CAD build for the part. Positions are in the model's coordinates, mm. A direction names the side the tool comes from. Round coordinates to 2 decimals unless told otherwise and drop trailing zeros. Loops run counter-clockwise (first coordinate to the right, second up) from the corner with the lowest first, then second, coordinate; pieces in that order, holes last.
from build123d import *

# Parameters (mm, degrees)
EXTRUDE_1_DEPTH     = 0.8
SKETCH_2_R          = 1.65
EXTRUDE_2_DEPTH     = 3.18
EXTRUDE_START       = 0.8
EXTRUDE_3_DEPTH     = 0.8
SKETCH_5_R          = 0.81
CUT_EXTRUDE_1_DEPTH = 4.8


with BuildPart() as part:
    # 草图1 → 凸台-拉伸1 (new body)
    with BuildSketch(Plane.XY):
        with BuildLine():
            ThreePointArc((1.190625, 2.753618004), (-3, 0), (1.190625, -2.753618004))
            ThreePointArc((1.190625, -2.753618004), (3.175, -2.342981343), (5.159375, -2.753618004))
            ThreePointArc((5.159375, -2.753618004), (9.35, 0), (5.159375, 2.753618004))
            ThreePointArc((5.159375, 2.753618004), (3.175, 2.342981343), (1.190625, 2.753618004))
        make_face()
    extrude(amount=EXTRUDE_1_DEPTH)

    # 草图2 → 凸台-拉伸2 (add)
    with BuildSketch(Plane(origin=(0, 0, 0), x_dir=(-1, 0, 0), z_dir=(0, 0, -1))):
        with Locations(Location((-6.35, 0, 0), (0, 0, 180))):
            Circle(SKETCH_2_R)
        with Locations(Location((0, 0, 0), (0, 0, 180))):
            Circle(SKETCH_2_R)
    extrude(amount=EXTRUDE_2_DEPTH)

    # 草图3 → 凸台-拉伸3 (add)
    with BuildSketch(Plane(origin=(0, 0, -3.18), x_dir=(-1, 0, 0), z_dir=(0, 0, -1)).offset(EXTRUDE_START)):
        with BuildLine():
            ThreePointArc((-1.190625, -2.753618004), (-3.175, -2.342981343), (-5.159375, -2.753618004))
            ThreePointArc((-5.159375, -2.753618004), (-9.35, 0), (-5.159375, 2.753618004))
            ThreePointArc((-5.159375, 2.753618004), (-3.175, 2.342981343), (-1.190625, 2.753618004))
            ThreePointArc((-1.190625, 2.753618004), (3, 0), (-1.190625, -2.753618004))
        make_face()
    extrude(amount=-EXTRUDE_3_DEPTH)

    # 草图5 → 切除-拉伸1 (cut)
    with BuildSketch(Plane(origin=(0, 0, -3.98), x_dir=(-1, 0, 0), z_dir=(0, 0, -1))):
        with Locations((-6.35, 0)):
            Circle(SKETCH_5_R)
        Circle(SKETCH_5_R)
    extrude(amount=-CUT_EXTRUDE_1_DEPTH, mode=Mode.SUBTRACT)


solid = part.part
Item 1: 3-axis set-ups, long thin cutter, end or side, ignore diameter. For faces 5 (the flat face through (3, 0, 0)), 6 (the cylindrical face through (-3, 0.1, -3.6)): which of +Z, -Z, +X, -X, +Y, -Y reach the whole face in a straight line?
Verdict:
face 5: none
face 6: +Z, -Z
Item 2: Flat gauge pins, fed straight in: P1, Ø1.3, axis at x = 0, y = 0, coming from the +Z side; P2, Ø1, axis at x = 6, z = -2, coming from the +Y side. Where does each tip first touch, or does it go through?
Verdict:
P1: passes through
P2: stops at y = 1.65
Item 3: Cut at D-D (z = -0.85). List the corners of the cut face in (x, y).
Verdict:
outline: circle Ø3.3 at (0, 0); circle Ø3.3 at (6.35, 0); hole circle Ø1.62 at (0, 0); hole circle Ø1.62 at (6.35, 0)
Item 4: Mould opens along Z. For faces 1 (the flat face through (3, 0, -3.18)), 2 (the flat face through (3, 0, 0.8)), 3 (the cylindrical face through (4.7, -0.07, -1.57)), 4 (the cylindrical face through (5.577, 0.243, -1.623)) say: released by +Z, released by -Z, zero draft, split by the parting line, or undercut.
Verdict:
face 1: undercut
face 2: released by +Z
face 3: undercut
face 4: zero draft
Item 5: Cut at A-A (y = 0). List the corners of the cut face in (x, z).
Verdict:
outline: (-3, -3.98) - (-0.81, -3.98) - (-0.81, 0.8) - (-3, 0.8) - (-3, 0) - (-1.65, 0) - (-1.65, -3.18) - (-3, -3.18) - close; (0.81, -3.98) - (5.54, -3.98) - (5.54, 0.8) - (0.81, 0.8) - close; (7.16, -3.98) - (9.35, -3.98) - (9.35, -3.18) - (8, -3.18) - (8, 0) - (9.35, 0) - (9.35, 0.8) - (7.16, 0.8) - close; hole (1.65, -3.18) - (4.7, -3.18) - (4.7, 0) - (1.65, 0) - close
Item 6: Wall check: L1, parallel to Z at x = 6.25, y = -2; L2, parallel to Y at x = 0, z = -1.35; L3, parallel to X at y = -0.5, z = -1.2. Give the ranges that are in metal, low to high.
Verdict:
L1: z = -3.98 to -3.18, 0 to 0.8
L2: y = -1.65 to -0.81, 0.81 to 1.65
L3: x = -1.57 to -0.64, 0.64 to 1.57, 4.78 to 5.71, 6.99 to 7.92
Item 7: Cut at C-C (z = -3.3). List the corners of the cut face in (x, y) (3 decimals), plus the area to 3 significant figures.
Verdict:
outline: (1.191, -2.754) arc R5 cw to (5.159, -2.754) arc R3 ccw (long way) to (5.159, 2.754) arc R5 cw to (1.191, 2.754) arc R3 ccw (long way) to start; hole circle Ø1.62 at (0, 0); hole circle Ø1.62 at (6.35, 0)
area: 57.7 mm2
Item 8: Cut at B-B (x = 0). List the corners of the cut face in (y, z), plus the area to 3 significant figures.
Verdict:
outline: (-3, -3.98) - (-0.81, -3.98) - (-0.81, 0.8) - (-3, 0.8) - (-3, 0) - (-1.65, 0) - (-1.65, -3.18) - (-3, -3.18) - close; (0.81, -3.98) - (3, -3.98) - (3, -3.18) - (1.65, -3.18) - (1.65, 0) - (3, 0) - (3, 0.8) - (0.81, 0.8) - close
area: 12.4 mm2
